Autodesk Inventor part; units mm, degrees
ref_plane "YZ Plane" through (0, 0, 0) normal (1, 0, 0) x (0, 1, 0)
ref_plane "XZ Plane" through (0, 0, 0) normal (0, 1, 0) x (-1, 0, 0)
ref_plane "XY Plane" through (0, 0, 0) normal (0, 0, 1) x (1, 0, 0)
sketch "Sketch1" plane through (0, 0, 0) normal (0, 0, 1) x (1, 0, 0)
  line L0 (-54.5, -12.5) -> (154.5, -12.5)
  line L1 (154.5, -12.5) -> (154.5, 12.5)
  line L2 (154.5, 12.5) -> (-54.5, 12.5)
  line L3 (-54.5, 12.5) -> (-54.5, -12.5)
  line L4 (-54.5, -12.5) -> (154.5, 12.5) construction
  line L5 (154.5, -12.5) -> (-54.5, 12.5) construction
  line L6 (149.5, 192.0914) -> (-150.5, 192.0914)
  line L7 (205, 191) -> (-105, 191)
  point P0 (50, 0)
  point P1 (50, 0)
  point P2 (50, 0)
  point P3 (50, 191)
  dimension "d0" = 25
  dimension "d1" = 209
extrude "Plate1" add sketch "Sketch1" along normal blind 2
sketch "Sketch2" plane through (153.5, -12.5, 0.2679) normal (0.5, 0, 0.8660254) x (0, 1, 0)
  line L0 (25, 0) -> (0, 0)
  line L1 (0, 0) -> (0, -25)
  line L2 (0, -25) -> (25, -25)
  line L3 (25, -25) -> (25, 0)
edge flange "Flange1" height 25 angle 30 thickness 2 bend radius 2 thickness toward (0.5, 0, 0.8660254) relief tear relief width 2 relief depth 1 corner gap 2 corner form 0 edges at (154.5, 0, 0) (-54.5, 0, 0) wall of the first edge with corners at (153.5, 12.5, 0.2679) (153.5, -12.5, 0.2679) (175.1506, -12.5, -12.2321) (175.1506, 12.5, -12.2321)
bend "Bend1"
corner "Corner1"
sketch "Sketch3" plane through (175.1506, 12.5, -10.2321) normal (0, 0, -1) x (-1, 0, 0)
  line L0 (0, -25) -> (0, 0)
  line L1 (0, 0) -> (-29, 0)
  line L2 (-29, 0) -> (-29, -25)
  line L3 (-29, -25) -> (0, -25)
edge flange "Flange2" height 29 angle 30 thickness 2 bend radius 2 thickness toward (0, 0, -1) relief tear relief width 2 relief depth 1 corner gap 2 corner form 0 edges at (176.1506, 0, -10.5) (-76.1506, 0, -10.5) wall of the first edge with corners at (175.1506, -12.5, -10.2321) (175.1506, 12.5, -10.2321) (204.1506, 12.5, -10.2321) (204.1506, -12.5, -10.2321)
bend "Bend2"
corner "Corner2"
sketch "Sketch4" plane through (0, 0, 2) normal (0, 0, 1) x (1, 0, 0)
  line L0 (-14.5, 0) -> (-4.5, 0) construction
  line L1 (-14.5, -3.2) -> (-4.5, -3.2)
  line L2 (-4.5, 3.2) -> (-14.5, 3.2)
  arc A0 (-14.5, 3.2) -> (-14.5, -3.2) centre (-14.5, 0) ccw
  arc A1 (-4.5, -3.2) -> (-4.5, 3.2) centre (-4.5, 0) ccw
  line L3 (60.5, 0) -> (70.5, 0) construction
  line L4 (60.5, -3.2) -> (70.5, -3.2)
  line L5 (70.5, 3.2) -> (60.5, 3.2)
  arc A2 (60.5, 3.2) -> (60.5, -3.2) centre (60.5, 0) ccw
  arc A3 (70.5, -3.2) -> (70.5, 3.2) centre (70.5, 0) ccw
  circle A4 centre (-9.5, 0) radius 3
  circle A5 centre (65.5, 0) radius 2.3866
  point P0 (0, 0)
  point P1 (-9.5, 0)
  point P2 (65.5, 0)
  dimension "d23" = 3.2
  dimension "d24" = 3.2
  dimension "d25" = 10
  dimension "d26" = 10
extrude "Cut1" cut sketch "Sketch4" against normal blind 2 contours A0 L2 A1 L1 | A2 L5 A3 L4 | A4 | A5
sketch "Sketch5" plane through (-104.1506, -12.5, -10.2321) normal (0, 0, 1) x (1, 0, 0)
  line L0 (0, 25) -> (0, 0)
  line L1 (308.3013, 0) -> (308.3013, 25)
  circle A0 centre (300.8013, 12.5) radius 2.75
  circle A1 centre (7.5, 12.5) radius 2.75
  point P0 (104.1506, 12.5)
  point P1 (300.8013, 12.5)
  point P2 (0, 12.5)
  point P3 (308.3013, 12.5)
hole "Hole1" at (-96.6506, 0, -10.2321) at (196.6506, 0, -10.2321) direction (0, 0, -1) diameter 7 depth 2 tip angle 118
fillet "Corner Round1" radius 6 4 edges at (-104.1506, 12.5, -11.2321) (-104.1506, -12.5, -11.2321) (204.1506, 12.5, -11.2321) (204.1506, -12.5, -11.2321)
equation "\"d27\" = Thickness"
equation "\"d36\" = Thickness"
equation "\"d3\" = BendReliefWidth"
equation "\"d4\" = BendReliefDepth"
equation "\"d5\" = MinimumRemnant"
equation "\"d6\" = BendRadius"
equation "\"d9\" = BendRadius"
equation "\"d10\" = CornerReliefSize"
equation "\"d11\" = GapSize"
equation "\"d12\" = JacobiRadiusSize"
equation "\"d13\" = BendReliefWidth"
equation "\"d14\" = BendReliefDepth"
equation "\"d15\" = MinimumRemnant"
equation "\"d16\" = BendRadius"
equation "\"d19\" = BendRadius"
equation "\"d20\" = CornerReliefSize"
equation "\"d21\" = GapSize"
equation "\"d22\" = JacobiRadiusSize"
equation "\"BendRadius\" = Thickness"
equation "\"BendReliefWidth\" = Thickness"
equation "\"BendReliefDepth\" = 0.5 * Thickness"
equation "\"CornerReliefSize\" = 4 * Thickness"
equation "\"MinimumRemnant\" = 2 * Thickness"
equation "\"TransitionRadius\" = BendRadius"
equation "\"JacobiRadiusSize\" = BendRadius"
equation "\"GapSize\" = Thickness"
equation "\"d2\" = BendRadius"
Geometry check sheet. Reference: the model listing, model coordinates, mm. A direction names the side the tool comes from. Round coordinates to 2 decimals unless told otherwise and drop trailing zeros. Loops run counter-clockwise (first coordinate to the right, second up) from the corner with the lowest first, then second, coordinate; pieces in that order, holes last.
Item 1: Cross-section at C-C on x = 163.5. Record the boundary of the cut face in (y, z).
Item 2: Cross-section at B-B on x = 77. Record the boundary of the cut face in (y, z).
Item 3: Mould release check, pull along X, two halves, no side actions. Record for faces 1 (the flat face through (49, 0, 0)), 2 (the cylindrical face through (-102.44, 10.696, -11.246)), 3 (the cylindrical face through (202.44, -10.696, -11.246)): pulls with the +X half, pulls with the -X half, needs draft (parallel to the pull), parting line crosses it, or undercut.
Item 4: Access from +Z, -Z, +X, -X, +Y, -Y to the whole of each face (thin tool, end or side, straight path). Record for faces 4 (the flat face through (-64.187, 0.175, -5.902)), 5 (the flat face through (-90, 0, -10.232)), 6 (the cylindrical face through (-93.234, 0.759, -11.246)), 7 (the flat face through (190, 0, -10.232)).
Item 5: Cross-section at A-A on z = -6. Record the boundary of the cut face in (x, y).
Item 6: Gauge pin test, flat ends, axial feed: pin 1 (7.5 mm diameter, centred on x = 49, y = 1.5, fed in from -Z); pin 2 (2 mm diameter, centred on x = -53, y = -2, fed in from -Z); pin 3 (1.5 mm diameter, centred on y = 7, z = -7.5, fed in from -X). Record the tip position at first contact, or that the pin passes through.
Item 7: Thickness scan on line 1 (X direction, y = 0, z = -10.8); line 2 (X direction, y = 0, z = -11.4); line 3 (Z direction, x = -10, y = 7). Record the ranges inside material, lowest first.
Answer sheet:
1. outline: (-12.5, -5.51) - (12.5, -5.51) - (12.5, -3.2) - (-12.5, -3.2) - close
2. outline: (-12.5, 0) - (12.5, 0) - (12.5, 2) - (-12.5, 2) - close
3. face 1: undercut
3. face 2: pulls with the -X half
3. face 3: pulls with the +X half
4. face 4: -Z, +Y, -Y
4. face 5: +Z, -X, +Y, -Y
4. face 6: +Z, -Z
4. face 7: +Z, +X, +Y, -Y
5. outline: (-68.36, -12.5) - (-64.36, -12.5) - (-64.36, 12.5) - (-68.36, 12.5) - close; (164.36, -12.5) - (168.36, -12.5) - (168.36, 12.5) - (164.36, 12.5) - close
6. pin 1: stops at z = 0
6. pin 2: stops at z = -0.08
6. pin 3: stops at x = -72.25
7. line 1: x = -104.15 to -100.15, -93.15 to -72.67, 172.67 to 193.15, 200.15 to 204.15
7. line 2: x = -104.15 to -100.15, -93.15 to -73.71, 173.71 to 193.15, 200.15 to 204.15
7. line 3: z = 0 to 2
